```python
from build123d import *

# Parameters (mm, degrees)
F1_DEPTH = 8
F2_SIZE2 = 14.99999
F2_SIZE  = 3.99999
F3_SIZE2 = 4
F3_SIZE  = 15
F5_DEPTH = 50


# Not quite as in the source:
# - a fillet or chamfer is up to 0.001 mm smaller than in the source, because OpenCascade refuses the exact size


with BuildPart() as f1:
    # F0 (on Top) → F1 (new body)
    with BuildSketch(Plane.XY):
        Polygon((-126, 0), (0, 0), (0, 40), (-150, 40), align=None)
    extrude(amount=F1_DEPTH)

    # F2 (size 4 and 15 in the source; OpenCascade refuses exactly that, so slightly less here)
    f2_edges = [f1.edges().sort_by_distance(p)[0] for p in [
        (-63, 0, 8),
        (-138, 20, 8),
        (-63, 0, 0),
    ]]
    chamfer(f2_edges, length=F2_SIZE, length2=F2_SIZE2)

    # F3
    f3_edges = [f1.edges().sort_by_distance(p)[0] for p in [
        (-142.499997, 27.499995, 0),
    ]]
    f3_side = f1.faces().sort_by_distance((-71.315788, 27.719293, 0))[0]
    chamfer(f3_edges, length=F3_SIZE, length2=F3_SIZE2, reference=f3_side)

    # F4 (on face) → F5 (cut)
    with BuildSketch(Plane.YZ):
        Polygon((12.5, 6.5), (12.5, 4), (12.5, 1.5), (35, 1.5), (35, 6.5), align=None)
    extrude(amount=-F5_DEPTH, mode=Mode.SUBTRACT)


solid = f1.part
```
Source: CAD feature listing. Evaluate the final solid. Frame: model axes, mm. A direction names the side the tool comes from. Coordinates: 2 decimals unless noted, no trailing zeros. Return JSON: item names as keys, results as strings. Group by question number.
1) Set-up query: faces 1 (the face through (-25, 24, 6.5)), 2 (the face through (-74, 40, 4)). Return all of +Z, -Z, +X, -X, +Y, -Y with unobstructed straight access to the full face (end or side cutting, diameter ignored); none if empty.
2) Ray query, line 1 along Z through (x, y) = (-16.5, 15); line 2 along Z through (x, y) = (-65, 14); line 3 along Z through (x, y) = (-34.5, 11.5). Return the intervals inside material, ascending.
3) Contact query for a flat-ended pin moving along its axis: P1, Ø8, axis at x = -94.5, y = 9.5, coming from the -Z side. Output: stop coordinate, or through.
4) Mould query, pull axis Y, two halves, no side actions, for faces 3 (the face through (0, 24, 1)), 4 (the face through (-131.83, 24.08, 2.03)), 5 (the face through (-50, 24, 4)). Classes: +Y half, -Y half, draft (parallel to the pull), parting line (faces both ways), or undercut.
From the geometry:
{
 "1": {"face 1": "+X", "face 2": "+Z, -Z, +X, -X, +Y"},
 "2": {"line 1": "0 to 1.5, 6.5 to 8", "line 2": "0.27 to 7.73", "line 3": "0.93 to 7.07"},
 "3": {"P1": "z = 0.4"},
 "4": {"face 3": "draft", "face 4": "-Y half", "face 5": "undercut"}
}
